Work out the finished part from the listing and answer in its coordinate system (mm). A direction names the side the tool comes from. Give positions to 0.01 mm unless a question says otherwise; leave off trailing zeros. Loops run counter-clockwise (first coordinate to the right, second up) from the corner with the lowest first, then second, coordinate; pieces in that order, holes last. Notation, with made-up numbers: M 46,-22.5 L 86,-22.5 A20 ccw 86,-5.5 Z; hole C 65,44 d5. An arc over 180 degrees is marked long. Answer in a Markdown table with one row per item. Add a question column.
Autodesk Inventor part; units mm, degrees
ref_plane "Work Plane1" through (14.2875, 0, -1.5875) normal (1, 0, 0) x (0, 1, 0)
ref_plane "YZ Plane" through (0, 0, 0) normal (1, 0, 0) x (0, 1, 0)
ref_plane "XZ Plane" through (0, 0, 0) normal (0, 1, 0) x (-1, 0, 0)
sketch "Sketch1" plane through (0, 0, 0) normal (0, 0, 1) x (1, 0, 0)
  line L0 (0, 7.3323) -> (6.35, 3.6662)
  line L1 (6.35, 3.6662) -> (6.35, -3.6662)
  line L2 (6.35, -3.6662) -> (0, -7.3323)
  line L3 (0, -7.3323) -> (-6.35, -3.6662)
  line L4 (-6.35, -3.6662) -> (-6.35, 3.6662)
  line L5 (-6.35, 3.6662) -> (0, 7.3323)
  point P0 (0, 0)
  point P1 (0, 0)
  dimension "d0" = 12.7
extrude "Extrusion1" add sketch "Sketch1" along normal blind 25.4
sketch "Sketch2" plane through (0, 0, 0) normal (0, 0, -1) x (-1, 0, 0)
  circle A0 centre (0, 0) radius 15.875
  dimension "d3" = 31.75
extrude "Extrusion2" add sketch "Sketch2" along normal blind 1.5875
sketch "Sketch3" plane through (0, 0, -1.5875) normal (0, 0, -1) x (-1, 0, 0)
  circle A0 centre (0, 0) radius 14.2875
  dimension "d6" = 28.575
extrude "Extrusion3" add sketch "Sketch3" along normal blind 12.7
sketch "Sketch4" plane through (0, 0, -14.2875) normal (0, 0, -1) x (-1, 0, 0)
  circle A0 centre (0, 0) radius 14.2875 construction
hole "Hole1" at (0, 0, -14.2875) direction (0, 0, 1) diameter 4.9784 end through all
ref_plane "Work Plane1" through (14.2875, 0, -1.5875) normal (1, 0, 0) x (0, 1, 0)
sketch "Sketch5" plane through (14.2875, 0, -1.5875) normal (1, 0, 0) x (0, 1, 0)
  line L0 (-14.2875, -12.7) -> (14.2875, -12.7) construction
  line L1 (14.2875, 0) -> (-14.2875, 0) construction
  line L2 (14.2875, 0) -> (14.2875, -12.7) construction
  line L3 (14.2875, 0) -> (14.2875, -12.7) construction
  point P0 (0, 1.5875)
  point P1 (0, -6.35)
  point P2 (14.2875, -6.35)
hole "Hole2" at (14.2875, 0, -7.9375) direction (-1, 0, 0) diameter 3.683 depth 9.525
mirror "Mirror1" about plane through (0, 0, 0) normal (1, 0, 0) of "Hole2"
sketch "Sketch6" plane through (0, 0, 25.4) normal (0, 0, 1) x (1, 0, 0)
  circle A0 centre (0, 0) radius 6.35
  circle A1 centre (0, 0) radius 15.875 construction
  line L0 (6.35, 3.6662) -> (6.35, -3.6662) construction
  line L1 (6.35, -3.6662) -> (0, -7.3323) construction
  line L2 (0, -7.3323) -> (-6.35, -3.6662) construction
  line L3 (-6.35, -3.6662) -> (-6.35, 3.6662) construction
  line L4 (-6.35, 3.6662) -> (0, 7.3323) construction
  line L5 (0, 7.3323) -> (6.35, 3.6662) construction
  line L6 (0, 7.3323) -> (6.35, 3.6662)
  line L7 (6.35, 3.6662) -> (6.35, -3.6662)
  line L8 (6.35, -3.6662) -> (0, -7.3323)
  line L9 (0, -7.3323) -> (-6.35, -3.6662)
  line L10 (-6.35, -3.6662) -> (-6.35, 3.6662)
  line L11 (-6.35, 3.6662) -> (0, 7.3323)
extrude "Extrusion4" cut sketch "Sketch6" against normal blind 3.175 contours L7 L8 A0 | A0 L6 L7 | A0 L11 L6 | L8 L9 A0 | A0 L10 L11 | L9 L10 A0
sketch "Sketch7" plane through (0, 0, 0) normal (1, 0, 0) x (0, 1, 0)
  line L0 (14.2875, -1.5875) -> (14.2875, -14.2875) construction
  line L1 (14.2875, -14.2875) -> (2.4892, -14.2875) construction
  line L2 (2.4892, -14.2875) -> (2.4892, 25.4) construction
  line L3 (2.4892, 25.4) -> (6.35, 25.4) construction
  line L4 (6.35, 25.4) -> (6.35, 22.225) construction
  line L5 (6.35, 22.225) -> (7.3323, 22.225) construction
  line L6 (7.3323, 22.225) -> (7.3323, 0) construction
  line L7 (7.3323, 0) -> (15.875, 0) construction
  line L8 (15.875, 0) -> (15.875, -1.5875) construction
  line L9 (15.875, -1.5875) -> (14.2875, -1.5875) construction
  line L10 (-15.875, 0) -> (-7.3323, 0) construction
  line L11 (-7.3323, 0) -> (-7.3323, 22.225) construction
  line L12 (-7.3323, 22.225) -> (-6.35, 22.225) construction
  line L13 (-6.35, 22.225) -> (-6.35, 25.4) construction
  line L14 (-6.35, 25.4) -> (-2.4892, 25.4) construction
  line L15 (-2.4892, 25.4) -> (-2.4892, -14.2875) construction
  line L16 (-2.4892, -14.2875) -> (-14.2875, -14.2875) construction
  line L17 (-14.2875, -14.2875) -> (-14.2875, -1.5875) construction
  line L18 (-14.2875, -1.5875) -> (-15.875, -1.5875) construction
  line L19 (-15.875, -1.5875) -> (-15.875, 0) construction
  line L20 (6.35, 22.225) -> (6.0325, 22.225)
  line L21 (6.0325, 22.225) -> (6.0325, 23.1775)
  line L22 (6.0325, 23.1775) -> (6.35, 23.1775)
  line L23 (6.35, 23.1775) -> (6.35, 22.225)
  line L24 (0, -22.225) -> (0, 33.3375)
  point P0 (0, 0)
  dimension "d25" = 0.3175
  dimension "d26" = 0.9525
revolve "Revolution1" cut sketch "Sketch7" angle 360 about axis through (0, 0, -10) along (0, 0, 1)
sketch "Sketch8" plane through (0, 0, 25.4) normal (0, 0, 1) x (1, 0, 0)
  circle A0 centre (0, 0) radius 6.35
  circle A1 centre (0, 0) radius 2.4892
  circle A2 centre (0, 0) radius 15.875
  line L0 (6.35, 3.6662) -> (6.35, -3.6662)
  line L1 (6.35, -3.6662) -> (0, -7.3323)
  line L2 (0, -7.3323) -> (-6.35, -3.6662)
  line L3 (-6.35, -3.6662) -> (-6.35, 3.6662)
  line L4 (-6.35, 3.6662) -> (0, 7.3323)
  line L5 (0, 7.3323) -> (6.35, 3.6662)
extrude "Extrusion5" [suppressed]
properties part number "WCP-0102" material "Aluminum 6061"
(1) Which of the six approach directions +Z, -Z, +X, -X, +Y, -Y give full straight-line access (tool end or side, diameter ignored) to faces 4 (the face through (-13.63, -4.29, -7.85)), 5 (the face through (9.46, 1.8, -7.54)), 6 (the face through (-1.812, 5.754, 22.708)), 7 (the face through (-3.131, -5.525, 10.957))?
(2) Consider line 1 along Y through (x, z) = (0, 1); line 2 along Y through (x, z) = (0, -1) (3 decimals); line 3 along Z through (x, y) = (-7.25, 0). Determine where each line is inside the solid, lowest interval first. Write a range as from..to.
(3) Section B-B, the plane z = 17 is taken. Determine the outline of the cut face in (x, y), and give its area (3 significant figures).
(4) Each of these flat-tipped pins is pushed along its axis until it touches: P1, Ø8, axis at y = -3, z = 13, coming from the +X side; P2, Ø1.1, axis at y = 0, z = -9, coming from the -X side; P3, Ø10, axis at y = -6.5, z = 0, coming from the +X side. Where does it stop, or does it pass through?
(5) Section D-D, the plane x = 4 is taken. Determine the outline of the cut face in (y, z) (1 decimal).
(6) The mould has two halves that part along Y. Classify faces 1 (the face through (-4.762, 0, -8)), 2 (the face through (3.219, -5.474, 10.957)), 3 (the face through (11.83, 8.31, -1.588)): pulls with the +Y half, pulls with the -Y half, needs draft (parallel to the pull), parting line crosses it, or undercut.
(7) Section C-C, the plane x = 10.5 is taken. Determine the outline of the cut face in (y, z), and give its area (3 significant figures).
Numbers:
| question | item | result |
|---|---|---|
| 1 | face 4 | -Z |
| 1 | face 5 | +X |
| 1 | face 6 | none |
| 1 | face 7 | +Z, -X, -Y |
| 2 | line 1 | y = -7.33..-2.49, 2.49..7.33 |
| 2 | line 2 | y = -15.875..-2.489, 2.489..15.875 |
| 2 | line 3 | z = -14.29..-9.78, -6.1..0 |
| 3 | outline | M -6.35,-3.67 L 0,-7.33 L 6.35,-3.67 L 6.35,3.67 L 0,7.33 L -6.35,3.67 Z; hole C 0,0 d4.98 |
| 3 | area | 120 mm² |
| 4 | P1 | stops at x = 6.35 |
| 4 | P2 | stops at x = -4.76 |
| 4 | P3 | stops at x = 15.8 |
| 5 | outline | M -15.4,-1.6 L -13.7,-1.6 L -13.7,-14.3 L 13.7,-14.3 L 13.7,-1.6 L 15.4,-1.6 L 15.4,0 L 5,0 L 5,22.2 L 4.5,22.2 L 4.5,23.2 L 4.9,23.2 L 4.9,25.4 L -4.9,25.4 L -4.9,23.2 L -4.5,23.2 L -4.5,22.2 L -5,22.2 L -5,0 L -15.4,0 Z |
| 6 | face 1 | undercut |
| 6 | face 2 | pulls with the -Y half |
| 6 | face 3 | needs draft |
| 7 | outline | M -11.91,-1.59 L -9.69,-1.59 L -9.69,-14.29 L 9.69,-14.29 L 9.69,-1.59 L 11.91,-1.59 L 11.91,0 L -11.91,0 Z; hole C 0,-7.94 d3.68 |
| 7 | area | 273 mm² |
